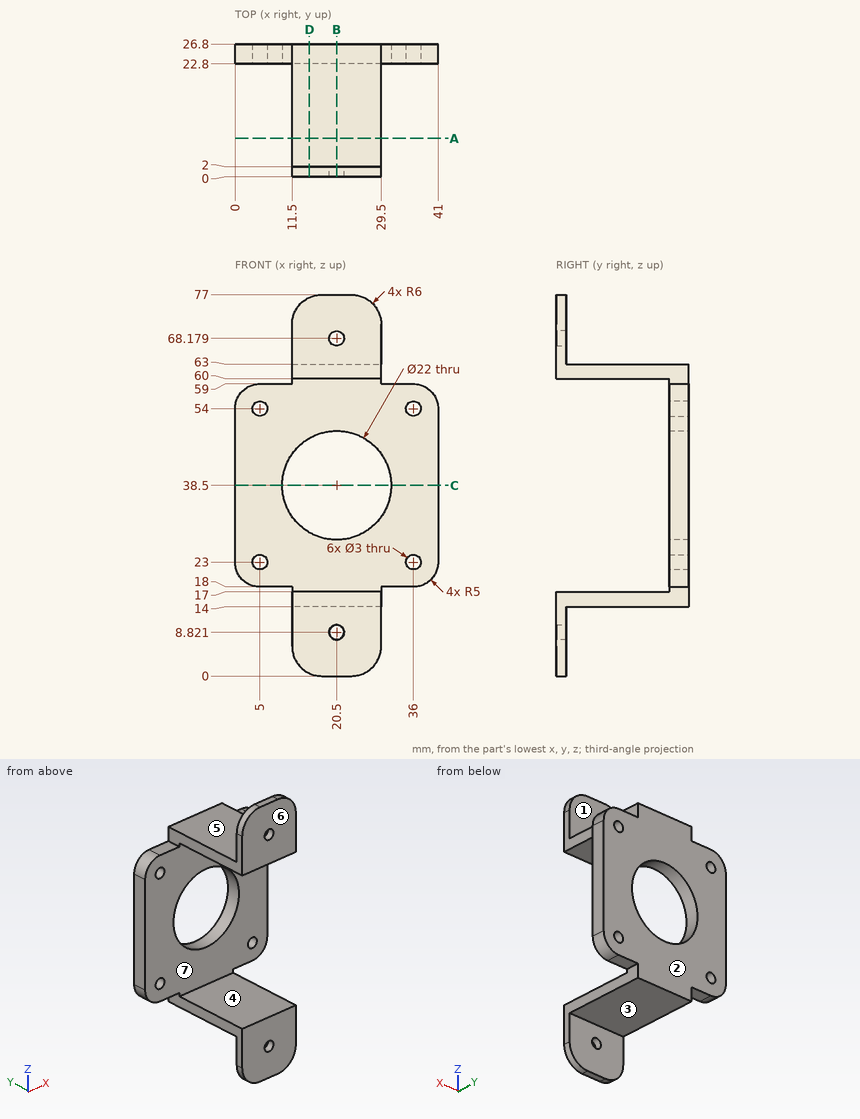
Answer from the drawing. Dimensions are ordinates in mm from the lowest x, y and z of the part. A direction names the side the tool comes from. Round coordinates to 2 decimals unless told otherwise and drop trailing zeros. Loops run counter-clockwise (first coordinate to the right, second up) from the corner with the lowest first, then second, coordinate; pieces in that order, holes last.
1) A cutting plane is placed at A-A on y = 7.75. Determine the outline of the cut face in (x, z).
Outcome:
outline: (11.5, 14) - (29.5, 14) - (29.5, 17) - (11.5, 17) - close; (11.5, 60) - (29.5, 60) - (29.5, 63) - (11.5, 63) - close
2) For the marked faces 1, 2, 3 and 4, determine the directions among +Z, -Z, +X, -X, +Y, -Y from which every point of the face is accessible in a straight line to the end or side of a thin tool.
Outcome:
face 1: +Z, +X, -X, +Y
face 2: +Z, -Z, +X, -X, +Y
face 3: -Z, +X, -X, +Y
face 4: +X, -X, -Y
3) A cutting plane is placed at D-D on x = 15. Determine the outline of the cut face in (y, z).
Outcome:
outline: (0, 0.55) - (2, 0.55) - (2, 14) - (26.8, 14) - (26.8, 28.97) - (22.8, 28.97) - (22.8, 17) - (0, 17) - close; (0, 60) - (22.8, 60) - (22.8, 48.03) - (26.8, 48.03) - (26.8, 63) - (2, 63) - (2, 76.45) - (0, 76.45) - close
4) Consider line 1 (X direction, y = 25.6, z = 54); line 2 (Y direction, x = 27, z = 70); line 3 (Y direction, x = 39, z = 21.5). Determine where each line is inside the solid, lowest interval first.
Outcome:
line 1: x = 0 to 3.5, 6.5 to 34.5, 37.5 to 41
line 2: y = 0 to 2
line 3: y = 22.8 to 26.8
5) A cutting plane is placed at B-B on x = 20.5. Determine the outline of the cut face in (y, z).
Outcome:
outline: (0, 0) - (2, 0) - (2, 7.32) - (0, 7.32) - close; (0, 10.32) - (2, 10.32) - (2, 14) - (26.8, 14) - (26.8, 27.5) - (22.8, 27.5) - (22.8, 17) - (0, 17) - close; (0, 60) - (22.8, 60) - (22.8, 49.5) - (26.8, 49.5) - (26.8, 63) - (2, 63) - (2, 66.68) - (0, 66.68) - close; (0, 69.68) - (2, 69.68) - (2, 77) - (0, 77) - close
6) A cutting plane is placed at C-C on z = 38.5. Determine the outline of the cut face in (x, y).
Outcome:
outline: (0, 22.8) - (9.5, 22.8) - (9.5, 26.8) - (0, 26.8) - close; (31.5, 22.8) - (41, 22.8) - (41, 26.8) - (31.5, 26.8) - close
7) Given P1, Ø4.5, axis at x = 9.5, y = 24.5, coming from the +Z side; P2, Ø13, axis at y = 10, z = 66.5, coming from the -X side; P3, Ø1.5, axis at x = 16.5, z = 56, coming from the -Y side; P4, Ø2.5, axis at x = 5, z = 23, coming from the +Y side, each flat-ended and moving along its own axis, determine where each tip first touches the part or whether it passes through.
Outcome:
P1: stops at z = 63
P2: stops at x = 11.5
P3: stops at y = 22.8
P4: passes through
8) For a pull along Z with two mould halves and no side action, classify the marked faces 5, 6 and 7 as released by +Z, released by -Z, zero draft, split by the parting line, or undercut.
Outcome:
face 5: released by +Z
face 6: zero draft
face 7: undercut
